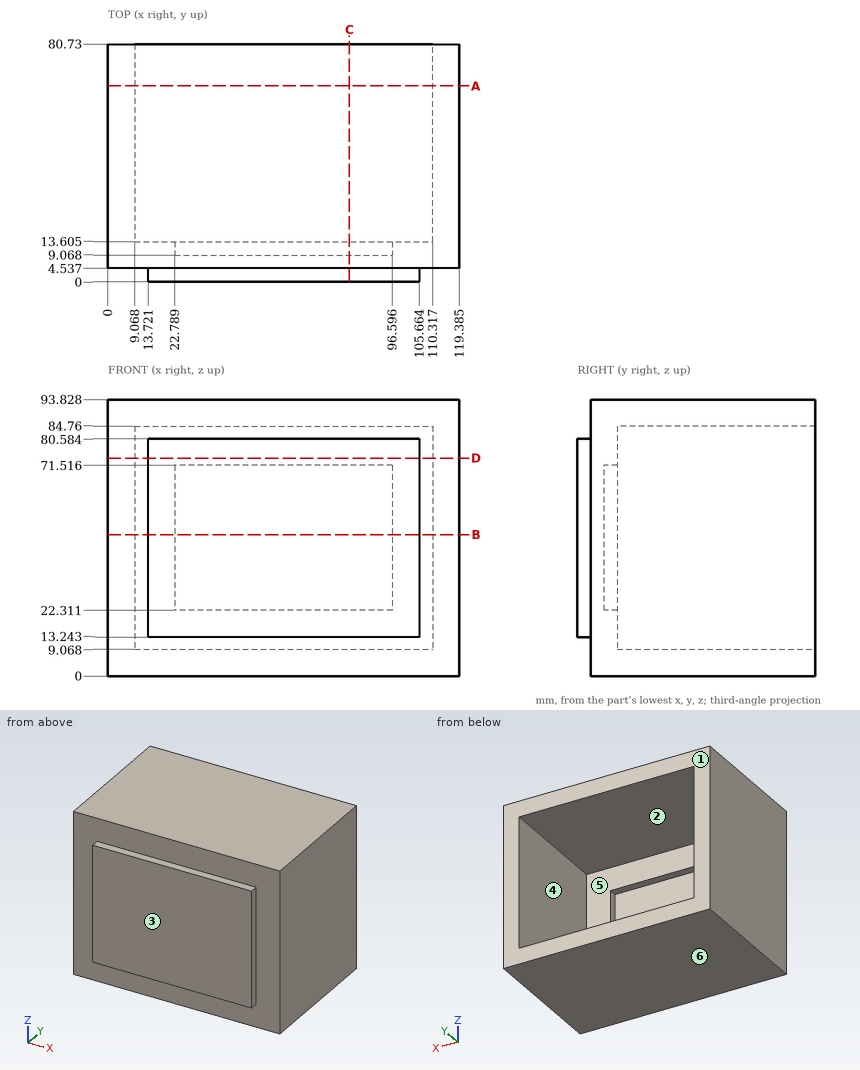
For this review, use the dimensioned drawing (mm, ordinates from the lowest corner) and the shaded views. A direction names the side the tool comes from. Round coordinates to 2 decimals unless told otherwise and drop trailing zeros. Order: outer loops, then holes, each group sorted by start corner. A loop starts at its lowest first (then second) coordinate and runs counter-clockwise, first axis right, second up. Notation, with made-up numbers: (54, 19) -> (105, 19) arc R6 cw to (105, 24) -> close; hole circle Ø6 at (71, 7.5). An arc over 180 degrees is marked (long way). Write item = value, one per line. Start each with the question number.
Item 1: For line 1 along X through (y, z) = (73.5, 66.5) (1 decimal); line 2 along Z through (x, y) = (29, 39.5); line 3 along X through (y, z) = (11.5, 35.5) (1 decimal), list the stretches that pass through material, from the lowest coordinate up.
Item 2: For the marked faces 1 and 2, list the 3-axis set-ups (+Z, -Z, +X, -X, +Y, -Y) from which the entire face can be reached by the end or side of a thin tool; tool diameter is ignored.
Item 3: Consider section B-B on z = 48. Write out the cut boundary in (x, y) (1 decimal).
Item 4: Mouldability with a two-part tool opening along Z and no side actions: class the marked faces 3, 4, 5 and 6 as released by +Z, released by -Z, zero draft, split by the parting line, or undercut.
Item 5: Consider section A-A on y = 66.5. Write out the cut boundary in (x, z) (1 decimal).
Item 6: Consider section D-D on z = 74. Write out the cut boundary in (x, y) (1 decimal), plus the area to 3 significant figures.
Item 7: Consider section C-C on x = 82. Write out the cut boundary in (y, z) (1 decimal), plus the area to 3 significant figures.
Item 8: Clearance check with flat-ended pins moving along their axes: pin 1 Ø1 at (x, z) = (83.5, 22.5) entering from +Y (1 decimal); pin 2 Ø1.4 at (y, z) = (3, 52) entering from +X; pin 3 Ø3.5 at (y, z) = (1.5, 55) entering from -X. State where each tip first meets the part, or that it passes through.
Conclusion:
q1.line_1 = 0 to 9.1, 110.3 to 119.4
q1.line_2 = 0 to 9.07, 84.76 to 93.83
q1.line_3 = 0 to 22.8, 96.6 to 119.4
q2.face_1 = +Z, -Z, +X, -X, +Y
q2.face_2 = +Y
q3.outline = (0, 4.5) -> (13.7, 4.5) -> (13.7, 0) -> (105.7, 0) -> (105.7, 4.5) -> (119.4, 4.5) -> (119.4, 80.7) -> (110.3, 80.7) -> (110.3, 13.6) -> (96.6, 13.6) -> (96.6, 9.1) -> (22.8, 9.1) -> (22.8, 13.6) -> (9.1, 13.6) -> (9.1, 80.7) -> (0, 80.7) -> close
q4.face_3 = zero draft
q4.face_4 = undercut
q4.face_5 = undercut
q4.face_6 = released by -Z
q5.outline = (0, 0) -> (119.4, 0) -> (119.4, 93.8) -> (0, 93.8) -> close; hole (9.1, 9.1) -> (110.3, 9.1) -> (110.3, 84.8) -> (9.1, 84.8) -> close
q6.outline = (0, 4.5) -> (13.7, 4.5) -> (13.7, 0) -> (105.7, 0) -> (105.7, 4.5) -> (119.4, 4.5) -> (119.4, 80.7) -> (110.3, 80.7) -> (110.3, 13.6) -> (9.1, 13.6) -> (9.1, 80.7) -> (0, 80.7) -> close
q6.area = 2,720 mm2
q7.outline = (0, 13.2) -> (4.5, 13.2) -> (4.5, 0) -> (80.7, 0) -> (80.7, 9.1) -> (13.6, 9.1) -> (13.6, 22.3) -> (9.1, 22.3) -> (9.1, 71.5) -> (13.6, 71.5) -> (13.6, 84.8) -> (80.7, 84.8) -> (80.7, 93.8) -> (4.5, 93.8) -> (4.5, 80.6) -> (0, 80.6) -> close
q7.area = 2,150 mm2
q8.pin_1 = 13.6
q8.pin_2 = 105.66
q8.pin_3 = 13.72
